```python
from build123d import *

# Parameters (mm, degrees)
SKETCH_1_R          = 2.5
EXTRUDE_587_DEPTH   = 5.6
SKETCH_2_OUTSIDE_W  = 296.81
SKETCH_2_OUTSIDE_H  = 295.654
SKETCH_2_OUTSIDE_R  = 3.736899617
CUT_EXTRUDE_1_DEPTH = 38
CUT_EXTRUDE_1_TAPER = 75
SKETCH_3_OUTSIDE_W  = 296.81
SKETCH_3_OUTSIDE_H  = 295.654
SKETCH_3_OUTSIDE_R  = 3.736899617
CUT_EXTRUDE_2_DEPTH = 38
CUT_EXTRUDE_2_TAPER = 75


with BuildPart() as part:
    # 草图1 → Extrude 587 (new body)
    with BuildSketch(Plane.XY):
        Polygon((2.1575, 3.736899617), (-2.1575, 3.736899617), (-4.315, 0), (-2.1575, -3.736899617), (2.1575, -3.736899617), (4.315, 0), align=None)
        Circle(SKETCH_1_R, mode=Mode.SUBTRACT)
    extrude(amount=EXTRUDE_587_DEPTH)

    # 草图2 outside → 切除-拉伸1 (cut)
    with BuildSketch(Plane(origin=(0, 0, 0), x_dir=(-1, 0, 0), z_dir=(0, 0, -1))):
        Rectangle(SKETCH_2_OUTSIDE_W, SKETCH_2_OUTSIDE_H)
        Circle(SKETCH_2_OUTSIDE_R, mode=Mode.SUBTRACT)
    extrude(amount=-CUT_EXTRUDE_1_DEPTH, taper=CUT_EXTRUDE_1_TAPER, mode=Mode.SUBTRACT)

    # 草图3 outside → 切除-拉伸2 (cut)
    with BuildSketch(Plane.XY.offset(5.6)):
        Rectangle(SKETCH_3_OUTSIDE_W, SKETCH_3_OUTSIDE_H)
        Circle(SKETCH_3_OUTSIDE_R, mode=Mode.SUBTRACT)
    extrude(amount=-CUT_EXTRUDE_2_DEPTH, taper=CUT_EXTRUDE_2_TAPER, mode=Mode.SUBTRACT)


solid = part.part
```
Could you check a few things on this model? Use its own coordinates, in mm. Round coordinates to 2 decimals unless told otherwise and drop trailing zeros. Write each loop counter-clockwise with the first axis right and the second up, starting at its lowest first coordinate (ties: lowest second). Pieces come first, ordered by that corner, then holes.
(1) If I drill on probe 1 along Y at (x, z) = (0, 3.4); probe 2 along X at (y, z) = (1.25, 1.85); probe 3 along Y at (x, z) = (0.5, 2.05), over which ranges is the centre line in solid material (lowest first)?
Findings below:
probe 1: y = -3.74 to -2.5, 2.5 to 3.74
probe 2: x = -3.59 to -2.17, 2.17 to 3.59
probe 3: y = -3.74 to -2.45, 2.45 to 3.74
(2) Suppose I cut it at A-A on z = 0.45. Write out the boundary of the cut face in (x, y) (1 decimal), and give its area (3 significant figures).
Findings below:
outline: (-4.3, 0) - (-2.2, -3.7) - (2.2, -3.7) - (4.3, 0) - (2.2, 3.7) - (-2.2, 3.7) - close; hole circle Ø5 at (0, 0)
area: 28.7 mm2
(3) Thinking about a two-plate mould opening in X: for faces 1 (the face through (-3.942, 0.01, 0.055)), 2 (the face through (3.942, 0.01, 5.545)), 3 (the face through (-0.54, -2.44, 2.76)), which applies, +X half, -X half, draft (parallel to the pull), parting line (faces both ways), or undercut?
Findings below:
face 1: -X half
face 2: +X half
face 3: undercut
